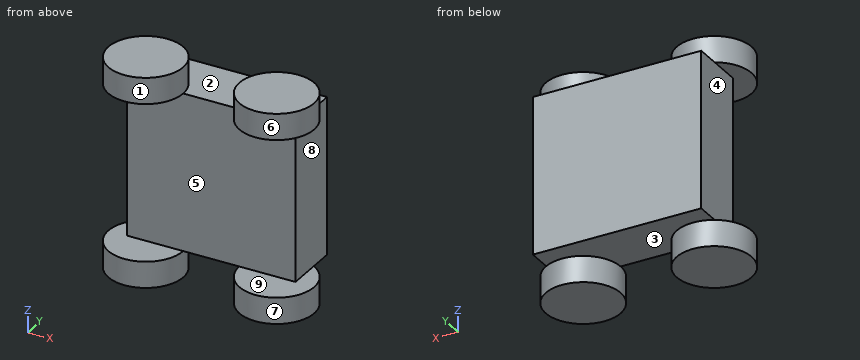
from build123d import *

# Parameters (mm, degrees)
SKETCH2_W           = 450
SKETCH2_H           = 420
BOSS_EXTRUDE1_DEPTH = 150
SKETCH3_R           = 100
BOSS_EXTRUDE2_DEPTH = 70


with BuildPart() as part:
    # Sketch2 → Boss-Extrude1 (new body)
    with BuildSketch(Plane(origin=(0, 0, 0), x_dir=(1, 0, 0), z_dir=(0, 1, 0))):
        Rectangle(SKETCH2_W, SKETCH2_H)
    extrude(amount=BOSS_EXTRUDE1_DEPTH)

    # Sketch3 → Boss-Extrude2 (add)
    with BuildSketch(Plane.XY.offset(210)):
        with Locations((-175, 0)):
            Circle(SKETCH3_R)
        with Locations(Location((175, 0, 0), (0, 0, 180))):
            Circle(SKETCH3_R)
    boss_extrude2 = extrude(amount=BOSS_EXTRUDE2_DEPTH)

    # Mirror1: Boss-Extrude2 across plane
    add(boss_extrude2.mirror(Plane.XY))


solid = part.part
Can you work these out from the model? Positions are in its coordinate system, mm. Face numbers are marked on the shaded views. A direction names the side the tool comes from. Give positions to 0.01 mm unless a question says otherwise; leave off trailing zeros. Write each loop counter-clockwise with the first axis right and the second up, starting at its lowest first coordinate (ties: lowest second). Pieces come first, ordered by that corner, then holes. Notation, with made-up numbers: M 4,14.5 L 21,14.5 A37 cw 21,52.5 Z; hole C 29,0 d6. An arc over 180 degrees is marked long. Answer in a Markdown table with one row per item. Add a question column.
Item 1: Imagine slicing it at B-B, the plane y = -54.5. Write out the boundary of the cut face in (x, z), plus the area to 3 significant figures.
Item 2: On a 3-axis mill with a long thin cutter (end or side, diameter ignored), from which of +Z, -Z, +X, -X, +Y, -Y can I reach the whole of each face in a straight line? I mean the marked faces 5, 6, 7, 8 and 9. Say none if no direction works.
Item 3: Imagine slicing it at A-A, the plane x = -175. Write out the boundary of the cut face in (y, z).
Item 4: We'd pull the mould along Z, two halves only. Please class the marked faces 1, 2, 3 and 4: released by +Z, released by -Z, zero draft, split by the parting line, or undercut.
Item 5: Imagine slicing it at C-C, the plane y = 61. Write out the boundary of the cut face in (x, z).
Item 6: For pin 1 Ø5 at (y, z) = (97, 135.5) entering from +X; pin 2 Ø3 at (x, z) = (63, 135) entering from -Y; pin 3 Ø1 at (x, y) = (-16.5, 2.5) entering from +Z, each with a flat end and sliding along its axis, tell me the tip position at first contact or that it passes through.
Item 7: Imagine slicing it at D-D, the plane z = -189. Write out the boundary of the cut face in (x, y), plus the area to 3 significant figures.
Item 8: Please list where these lines run through material, in increasing order: L1, parallel to Z at x = -207, y = -40.5; L2, parallel to X at y = -4.5, z = -236.5; L3, parallel to Y at x = 156, z = 82.
Evaluation:
| question | item | result |
|---|---|---|
| 1 | outline | M -258.84,-280 L -91.16,-280 L -91.16,-210 L -258.84,-210 Z; M -258.84,210 L -91.16,210 L -91.16,280 L -258.84,280 Z; M 91.16,-280 L 258.84,-280 L 258.84,-210 L 91.16,-210 Z; M 91.16,210 L 258.84,210 L 258.84,280 L 91.16,280 Z |
| 1 | area | 47,000 mm² |
| 2 | face 5 | +X, -X, -Y |
| 2 | face 6 | +Z |
| 2 | face 7 | -Z |
| 2 | face 8 | +X, +Y, -Y |
| 2 | face 9 | +X, -Y |
| 3 | outline | M -100,-280 L 100,-280 L 100,-210 L 150,-210 L 150,210 L 100,210 L 100,280 L -100,280 L -100,210 L 0,210 L 0,-210 L -100,-210 Z |
| 4 | face 1 | zero draft |
| 4 | face 2 | released by +Z |
| 4 | face 3 | released by -Z |
| 4 | face 4 | undercut |
| 5 | outline | M -254.24,-280 L -95.76,-280 L -95.76,-210 L 95.76,-210 L 95.76,-280 L 254.24,-280 L 254.24,-210 L 225,-210 L 225,210 L 254.24,210 L 254.24,280 L 95.76,280 L 95.76,210 L -95.76,210 L -95.76,280 L -254.24,280 L -254.24,210 L -225,210 L -225,-210 L -254.24,-210 Z |
| 6 | pin 1 | stops at x = 225 |
| 6 | pin 2 | stops at y = 0 |
| 6 | pin 3 | stops at z = 210 |
| 7 | outline | M -225,0 L 225,0 L 225,150 L -225,150 Z |
| 7 | area | 67,500 mm² |
| 8 | L1 | z = -280 to -210, 210 to 280 |
| 8 | L2 | x = -274.9 to -75.1, 75.1 to 274.9 |
| 8 | L3 | y = 0 to 150 |
